Verification items for the finished model (mm, model axes). A direction names the side the tool comes from. Round coordinates to 2 decimals unless told otherwise and drop trailing zeros. Order: outer loops, then holes, each group sorted by start corner. A loop starts at its lowest first (then second) coordinate and runs counter-clockwise, first axis right, second up. Notation, with made-up numbers: M 18.5,74 L 36.5,74 A15 ccw 36.5,90 Z; hole C -30,-24 d8. An arc over 180 degrees is marked long. Return JSON: item names as keys, results as strings. Group by question number.
from build123d import *

# Parameters (mm, degrees)
SKETCH_R        = 6
PAD_DEPTH       = 6
SKETCH002_R     = 3.5
POCKET_DEPTH    = 6.001
SKETCH001_R     = 4.5
POCKET001_DEPTH = 4
CHAMFER_SIZE    = 0.5
CHAMFER001_SIZE = 0.5
CHAMFER002_SIZE = 1


with BuildPart() as part:
    # Sketch → Pad (new body)
    with BuildSketch(Plane.XY):
        Circle(SKETCH_R)
    extrude(amount=PAD_DEPTH)

    # Sketch002 → Pocket (cut, through all)
    with BuildSketch(Plane(origin=(0, 0, 0), x_dir=(1, 0, 0), z_dir=(0, 0, -1))):
        Circle(SKETCH002_R)
    extrude(amount=-POCKET_DEPTH, mode=Mode.SUBTRACT)

    # Sketch001 → Pocket001 (cut)
    with BuildSketch(Plane(origin=(0, 0, 0), x_dir=(1, 0, 0), z_dir=(0, 0, -1))):
        Circle(SKETCH001_R)
    extrude(amount=-POCKET001_DEPTH, mode=Mode.SUBTRACT)

    # Chamfer
    chamfer_edges = [part.edges().sort_by_distance(p)[0] for p in [
        (-4.5, 0, 0),
    ]]
    chamfer(chamfer_edges, length=CHAMFER_SIZE)

    # Chamfer001
    chamfer001_edges = [part.edges().sort_by_distance(p)[0] for p in [
        (-3.5, 0, 4),
    ]]
    chamfer(chamfer001_edges, length=CHAMFER001_SIZE)

    # Chamfer002
    chamfer002_edges = [part.edges().sort_by_distance(p)[0] for p in [
        (-6, 0, 6),
    ]]
    chamfer(chamfer002_edges, length=CHAMFER002_SIZE)


solid = part.part
1. Access from +Z, -Z, +X, -X, +Y, -Y to the whole of each face (thin tool, end or side, straight path). Record for faces 4 (the face through (3.233, 1.341, 5.24)), 5 (the face through (-0.59, -4.46, 2.23)).
2. Cross-section at A-A (x = 0). Enter the section's corners in (y, z), plus the area to 3 significant figures.
3. Cross-section at C-C (z = 3.6). Enter the section's corners in (x, y).
4. Draft check along Y on faces 1 (the face through (-3, 3, 4)), 2 (the face through (-4, 4, 0)), 3 (the face through (-6, 0, 2)). Enter one of: +Y half, -Y half, draft (parallel to the pull), parting line (faces both ways), or undercut.
5. Go/stop test with flat-tipped pins: pin 1 (4 mm diameter, centred on x = 4.5, y = 3.5, fed in from -Z); pin 2 (7 mm diameter, centred on x = -0.5, y = -1, fed in from -Z); pin 3 (2 mm diameter, centred on y = -4, z = 1, fed in from -X); pin 4 (3 mm diameter, centred on y = 2, z = 4, fed in from +X). Record where each tip stops, or that it passes through.
6. Thickness scan on line 1 along Y through (x, z) = (-4, 2.5); line 2 along X through (y, z) = (-0.5, 0.75); line 3 along Z through (x, y) = (-4, -2). Record the ranges inside material, lowest first. Write a range as from..to.
Computed:
{
 "1": {"face 4": "+Z, -Z", "face 5": "-Z"},
 "2": {"outline": "M -6,0 L -5,0 L -4.5,0.5 L -4.5,4 L -4,4 L -3.5,4.5 L -3.5,6 L -5,6 L -6,5 Z; M 3.5,4.5 L 4,4 L 4.5,4 L 4.5,0.5 L 5,0 L 6,0 L 6,5 L 5,6 L 3.5,6 Z", "area": "20.5 mm²"},
 "3": {"outline": "C 0,0 d12; hole C 0,0 d9"},
 "4": {"face 1": "undercut", "face 2": "draft", "face 3": "parting line"},
 "5": {"pin 1": "stops at z = 0", "pin 2": "stops at z = 0.38", "pin 3": "stops at x = -5.2", "pin 4": "stops at x = 5.98"},
 "6": {"line 1": "y = -4.47..-2.06, 2.06..4.47", "line 2": "x = -5.98..-4.47, 4.47..5.98", "line 3": "z = 4..6"}
}
